For this review, take the finished solid that the model builds, in its own axes (mm). A direction names the side the tool comes from. Give positions to 0.01 mm unless a question says otherwise; leave off trailing zeros. Write each loop counter-clockwise with the first axis right and the second up, starting at its lowest first coordinate (ties: lowest second). Pieces come first, ordered by that corner, then holes. Notation, with made-up numbers: M -9.5,40 L 45.5,40 A16 cw 45.5,60 Z; hole C 57,10.5 d6. An arc over 180 degrees is marked long. Write item = value, one per line.
```python
from build123d import *

# Parameters (mm, degrees)
F0_W     = 101.6
F0_H     = 101.6
F0_W_2   = 88.9
F0_H_2   = 88.9
F1_DEPTH = 508
F3_DEPTH = 101.601
F4_R     = 5.08


with BuildPart() as f1:
    # F0 (on Top) → F1 (new body, symmetric)
    with BuildSketch(Plane.XY):
        Rectangle(F0_W, F0_H)
        Rectangle(F0_W_2, F0_H_2, mode=Mode.SUBTRACT)
    extrude(amount=F1_DEPTH, both=True)

    # F2 (on face) → F3 (cut, through all)
    with BuildSketch(Plane.XZ.offset(50.8)):
        Polygon((50.8, 508), (-50.8, 508), (50.8, 406.4), align=None)
        Polygon((50.8, -406.4), (-50.8, -508), (50.8, -508), align=None)
    extrude(amount=-F3_DEPTH, mode=Mode.SUBTRACT)

    # F4
    f4_edges = [f1.edges().sort_by_distance(p)[0] for p in [
        (-50.8, -50.8, 0),
        (50.8, -50.8, 0),
        (-50.8, 50.8, 0),
        (50.8, 50.8, 0),
        (44.45, 44.45, 0),
        (-44.45, 44.45, 0),
        (-44.45, -44.45, 0),
        (44.45, -44.45, 0),
    ]]
    fillet(f4_edges, radius=F4_R)


solid = f1.part
```
1. We need section A-A, the plane x = -30. Write out the cut boundary in (y, z).
Responses:
outline = M -50.8,-487.2 L -44.45,-487.2 L -44.45,487.2 L -50.8,487.2 Z; M 44.45,-487.2 L 50.8,-487.2 L 50.8,487.2 L 44.45,487.2 Z
2. Machinability: for faces 1 (the face through (-1, 50.8, 7)), 2 (the face through (-1, -44.45, 7)), which of the approach directions +Z, -Z, +X, -X, +Y, -Y give a long, thin tool a straight path to every point of the face, cutting with its end or side? Answer none if there is none.
Responses:
face_1 = +Z, -Z, +X, -X, +Y
face_2 = +Z, -Z
3. The part is to be moulded in two halves that separate along Y. For faces 3 (the face through (0.2, -45.4, -457)), 4 (the face through (-1, -50.8, 7)), 5 (the face through (44.45, -1, 6)), say which applies: +Y half, -Y half, draft (parallel to the pull), parting line (faces both ways), or undercut.
Responses:
face_3 = draft
face_4 = -Y half
face_5 = undercut
4. We need section B-B, the plane z = 364. Write out the cut boundary in (x, y), then the cut area to 3 significant figures.
Responses:
outline = M -50.8,-45.72 A5.08 ccw -45.72,-50.8 L 45.72,-50.8 A5.08 ccw 50.8,-45.72 L 50.8,45.72 A5.08 ccw 45.72,50.8 L -45.72,50.8 A5.08 ccw -50.8,45.72 Z; hole M -44.45,-39.37 A5.08 ccw -39.37,-44.45 L 39.37,-44.45 A5.08 ccw 44.45,-39.37 L 44.45,39.37 A5.08 ccw 39.37,44.45 L -39.37,44.45 A5.08 ccw -44.45,39.37 Z
area = 2,420 mm2
5. We need section C-C, the plane y = 3.5. Write out the cut boundary in (x, z).
Responses:
outline = M -50.8,-508 L -44.45,-501.65 L -44.45,501.65 L -50.8,508 Z; M 44.45,-412.75 L 50.8,-406.4 L 50.8,406.4 L 44.45,412.75 Z
6. For line 1 along X through (y, z) = (-9.5, -164.5); line 2 along Y through (x, z) = (44, -236.5), list the stretches that pass through material, from the lowest coordinate up. Write a range as from..to.
Responses:
line_1 = -50.8..-44.45, 44.45..50.8
line_2 = -50.8..-41.46, 41.46..50.8
